Geometry check sheet. Reference: the model listing, model coordinates, mm. Face numbers are marked on the shaded views. A direction names the side the tool comes from. Round coordinates to 2 decimals unless told otherwise and drop trailing zeros. Loops run counter-clockwise (first coordinate to the right, second up) from the corner with the lowest first, then second, coordinate; pieces in that order, holes last.
Solid Edge part; units mm, degrees
sketch "Sketch1" plane through (0, 0, 0) normal (0, 0, 1) x (1, 0, 0)
  line L0 (4.1, -3.45) -> (-4.1, -3.45)
  line L1 (-4.1, -3.45) -> (-4.1, 3.45)
  line L2 (-4.1, 3.45) -> (4.1, 3.45)
  line L3 (4.1, 3.45) -> (4.1, -3.45)
extrude "Protrusion1" add sketch "Sketch1" along normal blind 4.7
sketch "Sketch2" plane through (0, 0, 0) normal (0, 0, -1) x (1, 0, 0)
  circle A0 centre (-2, 1.25) radius 0.381
  circle A1 centre (0, 1.25) radius 0.381
  circle A2 centre (2, 1.25) radius 0.381
  circle A3 centre (2, -1.25) radius 0.381
  circle A4 centre (0, -1.25) radius 0.381
  circle A5 centre (-2, -1.25) radius 0.381
  circle A6 centre (-4.1, 0) radius 0.381
  circle A7 centre (4.1, 0) radius 0.381
extrude "ExtrudedProtrusion_2" add sketch "Sketch2" along normal blind 2.8
sketch "Sketch3" plane through (0, -3.45, 4.5593) normal (0, -1, 0) x (1, 0, 0)
  line L0 (2, -2.8593) -> (0, -2.8593)
  line L1 (0, -2.8593) -> (0, -0.8593)
  line L2 (0, -0.8593) -> (2, -0.8593)
  line L3 (2, -0.8593) -> (2, -2.8593)
extrude "ExtrudedProtrusion_3" add sketch "Sketch3" along normal blind 5.08
sketch "Sketch4" plane through (0, -3.45, 4.5593) normal (0, -1, 0) x (1, 0, 0)
  line L0 (-2, -0.8593) -> (-2, -2.8593)
  line L1 (-2, -2.8593) -> (0, -2.8593)
  line L2 (0, -2.8593) -> (0, -0.8593)
  line L3 (0, -0.8593) -> (-2, -0.8593)
extrude "ExtrudedCutout_1" cut sketch "Sketch4" against normal blind 2.54
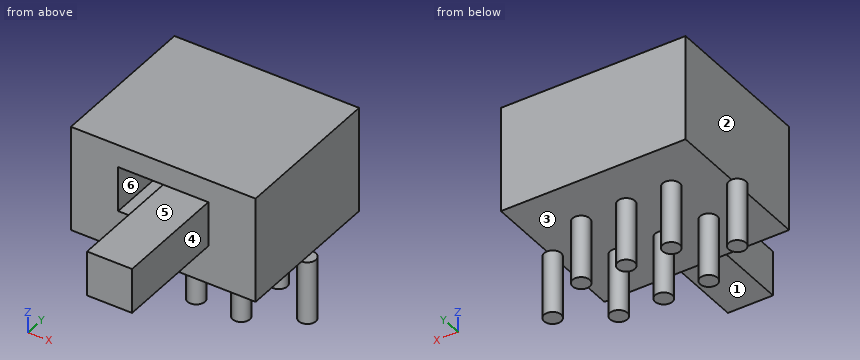
1) Gauge pin test, flat ends, axial feed: pin 1 (1.5 mm diameter, centred on x = 0.5, z = 0.5, fed in from -Y); pin 2 (0.6 mm diameter, centred on x = -1, z = 3, fed in from -Y); pin 3 (0.6 mm diameter, centred on y = -6, z = 3, fed in from -X). Record the tip position at first contact, or that the pin passes through.
Report:
pin 1: stops at y = -3.45
pin 2: stops at y = -0.91
pin 3: stops at x = 0
2) Scan lines: line 1 along X through (y, z) = (-7.25, 3); line 2 along Z through (x, y) = (-2.25, 2.5); line 3 along Y through (x, z) = (-3.25, 1.75). Record each from-to range of solid material in increasing order.
Report:
line 1: x = 0 to 2
line 2: z = 0 to 4.7
line 3: y = -3.45 to 3.45
3) Sectioned sample at C-C, the plane x = -1. Record the cut outline in (y, z), then the cut area to 4 significant figures.
Report:
outline: (-3.45, 0) - (3.45, 0) - (3.45, 4.7) - (-3.45, 4.7) - (-3.45, 3.7) - (-0.91, 3.7) - (-0.91, 1.7) - (-3.45, 1.7) - close
area: 27.35 mm2
4) Sectioned sample at A-A, the plane z = -0.5. Record the cut outline in (x, y).
Report:
outline: circle Ø0.76 at (-4.1, 0); circle Ø0.76 at (-2, -1.25); circle Ø0.76 at (-2, 1.25); circle Ø0.76 at (0, -1.25); circle Ø0.76 at (0, 1.25); circle Ø0.76 at (2, -1.25); circle Ø0.76 at (2, 1.25); circle Ø0.76 at (4.1, 0)
5) Mould release check, pull along X, two halves, no side actions. Record for the marked faces 1, 2 and 3: +X half, -X half, draft (parallel to the pull), parting line (faces both ways), or undercut.
Report:
face 1: draft
face 2: -X half
face 3: undercut
6) Sectioned sample at B-B, the plane y = -1.25. Record the cut outline in (x, z).
Report:
outline: (-4.1, 0) - (-2.38, 0) - (-2.38, -2.8) - (-1.62, -2.8) - (-1.62, 0) - (-0.38, 0) - (-0.38, -2.8) - (0.38, -2.8) - (0.38, 0) - (1.62, 0) - (1.62, -2.8) - (2.38, -2.8) - (2.38, 0) - (4.1, 0) - (4.1, 4.7) - (-4.1, 4.7) - close; hole (-2, 1.7) - (0, 1.7) - (0, 3.7) - (-2, 3.7) - close
7) Sectioned sample at D-D, the plane y = 1.25. Record the cut outline in (x, z).
Report:
outline: (-4.1, 0) - (-2.38, 0) - (-2.38, -2.8) - (-1.62, -2.8) - (-1.62, 0) - (-0.38, 0) - (-0.38, -2.8) - (0.38, -2.8) - (0.38, 0) - (1.62, 0) - (1.62, -2.8) - (2.38, -2.8) - (2.38, 0) - (4.1, 0) - (4.1, 4.7) - (-4.1, 4.7) - close
8) Access from +Z, -Z, +X, -X, +Y, -Y to the whole of each face (thin tool, end or side, straight path). Record for the marked faces 4, 5 and 6.
Report:
face 4: +Z, -Z, +X, -Y
face 5: +Z, +X, -X, -Y
face 6: -Y
